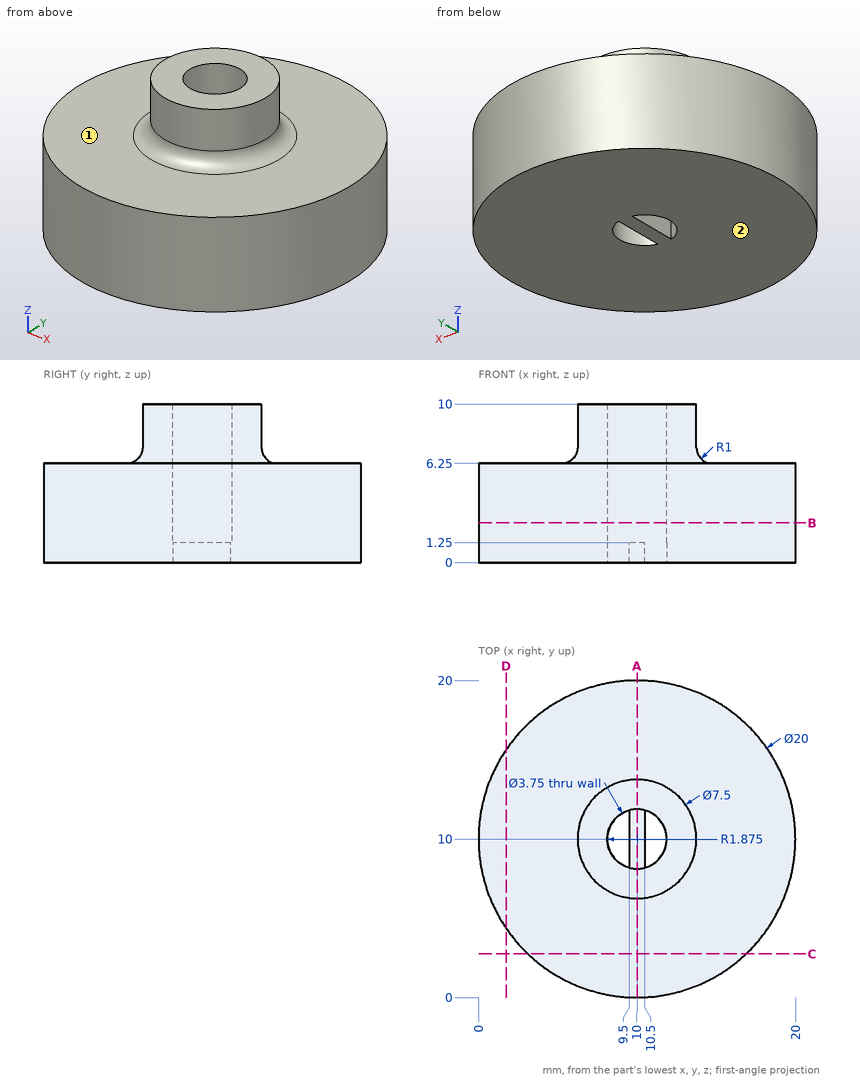
Geometry check sheet. Reference: drawing and pictorial views, mm from the part's lowest x, y, z. A direction names the side the tool comes from. Coordinates: 2 decimals unless noted, no trailing zeros. Write each loop counter-clockwise with the first axis right and the second up, starting at its lowest first coordinate (ties: lowest second). Pieces come first, ordered by that corner, then holes. Notation, with made-up numbers: (40, -16.75) -> (63, -16.75) arc R5 cw to (63, -12.75) -> close; hole circle Ø1 at (38, -16.5). An arc over 180 degrees is marked (long way). Use a Markdown table: item, result.
1. Sectioned sample at D-D (x = 1.75). Enter the section's corners in (y, z).
Reported:
| item | result |
|---|---|
| outline | (4.35, 0) -> (15.65, 0) -> (15.65, 6.25) -> (4.35, 6.25) -> close |
2. Scan lines: line 1 along Y through (x, z) = (10, 1.5) (3 decimals); line 2 along Z through (x, y) = (4, 8.5); line 3 along Y through (x, z) = (9.5, 5.25). Record each from-to range of solid material in increasing order.
Reported:
| item | result |
|---|---|
| line 1 | y = 0 to 8.125, 11.875 to 20 |
| line 2 | z = 0 to 6.25 |
| line 3 | y = 0.01 to 8.19, 11.81 to 19.99 |
3. Sectioned sample at B-B (z = 2.5). Enter the section's corners in (x, y) (3 decimals).
Reported:
| item | result |
|---|---|
| outline | circle Ø20 at (10, 10); hole circle Ø3.75 at (10, 10) |
4. Sectioned sample at C-C (y = 2.75). Enter the section's corners in (x, z), plus the area to 3 significant figures.
Reported:
| item | result |
|---|---|
| outline | (3.11, 0) -> (16.89, 0) -> (16.89, 6.25) -> (3.11, 6.25) -> close |
| area | 86.1 mm2 |
5. Go/stop test with flat-tipped pins: pin 1 Ø4 at (x, y) = (16, 6.5) entering from +Z; pin 2 Ø3 at (x, y) = (10, 10) entering from +Z; pin 3 Ø1.5 at (y, z) = (6, 3.5) entering from -X. Record where each tip stops, or that it passes through.
Reported:
| item | result |
|---|---|
| pin 1 | stops at z = 6.25 |
| pin 2 | stops at z = 1.25 |
| pin 3 | stops at x = 0.54 |
6. Sectioned sample at A-A (x = 10). Enter the section's corners in (y, z) (3 decimals).
Reported:
| item | result |
|---|---|
| outline | (0, 0) -> (20, 0) -> (20, 6.25) -> (14.75, 6.25) arc R1 cw to (13.75, 7.25) -> (13.75, 10) -> (11.875, 10) -> (11.875, 1.25) -> (8.125, 1.25) -> (8.125, 10) -> (6.25, 10) -> (6.25, 7.25) arc R1 cw to (5.25, 6.25) -> (0, 6.25) -> close |
7. Tool access check on the marked faces 1 and 2. Record the directions out of +Z, -Z, +X, -X, +Y, -Y that give a thin tool (end or side, any length) a straight path to the whole face; none if there is none.
Reported:
| item | result |
|---|---|
| face 1 | +Z |
| face 2 | -Z, +X, -X, +Y, -Y |
